from build123d import *

# Parameters (mm, degrees)
SKETCH3_W                      = 31.148374891
SKETCH3_H                      = 19.837641971
BOSS_EXTRUDE1_DEPTH            = 6.35
SKETCH4_R                      = 3.175
CUT_EXTRUDE1_DEPTH             = 9.525
SKETCH5_R                      = 3.175
CUT_EXTRUDE5_DEPTH             = 9.525
CUT_EXTRUDE5_DIRECTION_2_REACH = 33.299
SKETCH6_R                      = 3.175
CUT_EXTRUDE6_DEPTH             = 9.525


with BuildPart() as part:
    # Sketch3 → Boss-Extrude1 (new, symmetric)
    with BuildSketch(Plane.XY):
        with Locations((15.574187446, -9.918820986)):
            Rectangle(SKETCH3_W, SKETCH3_H)
    extrude(amount=BOSS_EXTRUDE1_DEPTH, both=True)

    # Sketch4 → Cut-Extrude1 (cut)
    with BuildSketch(Plane.ZY):
        with Locations(Location((0, -6.35, 0), (0, 0, 270))):
            Circle(SKETCH4_R)
    extrude(amount=-CUT_EXTRUDE1_DEPTH, mode=Mode.SUBTRACT)

    # Sketch5 → Cut-Extrude5 (cut)
    with BuildSketch(Plane(origin=(7.787093723, -19.837641971, 0), x_dir=(-0.8660254037844382, 0.500000000000001, 0), z_dir=(-0.500000000000001, -0.8660254037844382, 0))):
        with Locations(Location((0, 0, 0), (0, 0, 180))):
            Circle(SKETCH5_R)
    cut_extrude5 = extrude(amount=-CUT_EXTRUDE5_DEPTH, mode=Mode.SUBTRACT)

    # Sketch5 → Cut-Extrude5 direction 2 (cut, up to next)
    with BuildSketch(Plane(origin=(7.787093723, -19.837641971, 0), x_dir=(-0.8660254037844382, 0.500000000000001, 0), z_dir=(-0.500000000000001, -0.8660254037844382, 0)), mode=Mode.PRIVATE) as cut_extrude5_direction_2_sk1:
        with Locations(Location((0, 0, 0), (0, 0, 180))):
            Circle(SKETCH5_R)
    cut_extrude5_direction_2_tool1 = extrude(cut_extrude5_direction_2_sk1.sketch, amount=CUT_EXTRUDE5_DIRECTION_2_REACH, mode=Mode.PRIVATE) & part.part
    cut_extrude5_direction_2 = cut_extrude5_direction_2_tool1.solids().sort_by_distance((7.787094, -19.837642, 0))[0]
    add(cut_extrude5_direction_2, mode=Mode.SUBTRACT)

    # Sketch6 → Cut-Extrude6 (cut)
    with BuildSketch(Plane(origin=(0, 0, 6.35), x_dir=(-1, 0, 0), z_dir=(0, 0, -1))):
        with Locations(Location((-15.574187445, -6.35, 0), (0, 0, 180))):
            Circle(SKETCH6_R)
    extrude(amount=CUT_EXTRUDE6_DEPTH, mode=Mode.SUBTRACT)

    # Mirror1: Cut-Extrude5, Cut-Extrude5 direction 2 across plane
    add(cut_extrude5.mirror(Plane.ZY.offset(-15.574187445)), mode=Mode.SUBTRACT)
    add(cut_extrude5_direction_2.mirror(Plane.ZY.offset(-15.574187445)), mode=Mode.SUBTRACT)


solid = part.part
Geometry check sheet. Reference: the model listing, model coordinates, mm. A direction names the side the tool comes from. Coordinates: 2 decimals unless noted, no trailing zeros. Order: outer loops, then holes, each group sorted by start corner. A loop starts at its lowest first (then second) coordinate and runs counter-clockwise, first axis right, second up. Notation, with made-up numbers: (15, 24.5) -> (71, 24.5) arc R24 cw to (71, 57.5) -> close; hole circle Ø5 at (0, -12.5). An arc over 180 degrees is marked (long way). Use a Markdown table: item, result. Add a question column.
1. Cross-section at A-A (z = 4). Enter the section's corners in (x, y) (3 decimals).
2. Cross-section at B-B (y = -3.75). Enter the section's corners in (x, z) (3 decimals).
3. Set-up check for faces 5 (the face through (12.511, -11.567, 0.044)), 6 (the face through (13.234, -8.496, 1.654)), 7 (the face through (4.7, -3.18, 0.14)): record each of +Z, -Z, +X, -X, +Y, -Y from which the full face is reachable in a straight line by a thin tool's end or side.
4. Go/stop test with flat-tipped pins: pin 1 Ø1.9 at (x, y) = (15.5, -6) entering from +Z (3 decimals); pin 2 Ø1.9 at (y, z) = (-7.5, 0.5) entering from -X (3 decimals); pin 3 Ø6 at (y, z) = (-7.5, -1.5) entering from -X. Record where each tip stops, or that it passes through.
5. Cross-section at D-D (y = -6.35). Enter the section's corners in (x, z) (3 decimals).
6. Mould release check, pull along Y, two halves, no side actions. Record for faces 1 (the face through (15, -19.838, 0)), 2 (the face through (9.525, -6, 0)), 3 (the face through (15, 0, 0)), 4 (the face through (0, -10, 0)): pulls with the +Y half, pulls with the -Y half, needs draft (parallel to the pull), parting line crosses it, or undercut.
7. Cross-section at C-C (z = 0.75). Enter the section's corners in (x, y) (3 decimals), and give its area (3 significant figures).
8. Material ranges on L1, parallel to X at y = -6.35, z = -1 (3 decimals); L2, parallel to Z at x = 22.5, y = -18.25; L3, parallel to X at y = -15, z = -1.5, recorded low to high.
Filled sheet:
| question | item | result |
|---|---|---|
| 1 | outline | (0, -19.838) -> (31.148, -19.838) -> (31.148, 0) -> (0, 0) -> close; hole circle Ø6.35 at (15.574, -6.35) |
| 2 | outline | (0, -6.35) -> (31.148, -6.35) -> (31.148, 6.35) -> (17.396, 6.35) -> (17.396, -3.175) -> (13.752, -3.175) -> (13.752, 6.35) -> (0, 6.35) -> (0, 1.822) -> (9.525, 1.822) -> (9.525, -1.822) -> (0, -1.822) -> close |
| 3 | face 5 | none |
| 3 | face 6 | +Z |
| 3 | face 7 | -X |
| 4 | pin 1 | z = -3.175 |
| 4 | pin 2 | x = 9.525 |
| 4 | pin 3 | x = 0 |
| 5 | outline | (0, -6.35) -> (31.148, -6.35) -> (31.148, 6.35) -> (18.749, 6.35) -> (18.749, -3.175) -> (12.399, -3.175) -> (12.399, 6.35) -> (0, 6.35) -> (0, 3.175) -> (9.525, 3.175) -> (9.525, -3.175) -> (0, -3.175) -> close |
| 6 | face 1 | pulls with the -Y half |
| 6 | face 2 | undercut |
| 6 | face 3 | pulls with the +Y half |
| 6 | face 4 | needs draft |
| 7 | outline | (0, -19.838) -> (4.225, -19.838) -> (9.878, -10.046) -> (15.221, -13.131) -> (11.35, -19.838) -> (19.799, -19.838) -> (15.927, -13.131) -> (21.271, -10.046) -> (26.924, -19.838) -> (31.148, -19.838) -> (31.148, 0) -> (0, 0) -> (0, -3.265) -> (9.525, -3.265) -> (9.525, -9.435) -> (0, -9.435) -> close; hole circle Ø6.35 at (15.574, -6.35) |
| 7 | area | 410 mm2 |
| 8 | L1 | 9.525 to 12.399, 18.749 to 31.148 |
| 8 | L2 | -6.35 to -3.17, 3.17 to 6.35 |
| 8 | L3 | 0 to 7.35, 13.81 to 17.34, 23.8 to 31.15 |
